Geometry check sheet. Reference: the model listing, model coordinates, mm. A direction names the side the tool comes from. Give positions to 0.01 mm unless a question says otherwise; leave off trailing zeros. Order: outer loops, then holes, each group sorted by start corner. A loop starts at its lowest first (then second) coordinate and runs counter-clockwise, first axis right, second up.
from build123d import *

# Parameters (mm, degrees)
BOSS_EXTRUDE1_DEPTH                                 = 15
TAP_DRILL_FOR_M6_TAP1_D                             = 5
CBORE_FOR_M6_HEX_SOCKET_HEAD_CAP_SCREW1_D           = 6.6
CBORE_FOR_M6_HEX_SOCKET_HEAD_CAP_SCREW1_CBORE_D     = 11
CBORE_FOR_M6_HEX_SOCKET_HEAD_CAP_SCREW1_CBORE_DEPTH = 6.4
CHAMFER1_SIZE                                       = 0.5


with BuildPart() as part:
    # Sketch1 → Boss-Extrude1 (new body)
    with BuildSketch(Plane.XY):
        with BuildLine():
            Line((2.914096072, -75.45920495), (9.914096072, -75.45920495))
            ThreePointArc((9.914096072, -75.45920495), (12.742523197, -74.287632074), (13.914096072, -71.45920495))
            Line((13.914096072, -71.45920495), (13.914096072, 14.148669163))
            ThreePointArc((13.914096072, 14.148669163), (14.675300747, 17.975503486), (16.84302826, 21.219736974))
            Line((16.84302826, 21.219736974), (18.985163884, 23.361872598))
            ThreePointArc((18.985163884, 23.361872598), (22.229397372, 25.529600111), (26.056231696, 26.290804786))
            Line((26.056231696, 26.290804786), (26.414096072, 26.290804786))
            ThreePointArc((26.414096072, 26.290804786), (32.914096072, 32.790804786), (26.414096072, 39.290804786))
            Line((26.414096072, 39.290804786), (20.671455385, 39.290804786))
            ThreePointArc((20.671455385, 39.290804786), (16.844621061, 38.529600111), (13.600387573, 36.361872598))
            Line((13.600387573, 36.361872598), (1.84302826, 24.604513285))
            ThreePointArc((1.84302826, 24.604513285), (-0.324699253, 21.360279797), (-1.085903928, 17.533445473))
            Line((-1.085903928, 17.533445473), (-1.085903928, -71.45920495))
            ThreePointArc((-1.085903928, -71.45920495), (0.085668947, -74.287632074), (2.914096072, -75.45920495))
        make_face()
    extrude(amount=BOSS_EXTRUDE1_DEPTH)

    # Tap Drill for M6 Tap1 (through all)
    with Locations(Plane.XY.offset(15)):
        with Locations((26.414096072, 32.790804786)):
            Hole(TAP_DRILL_FOR_M6_TAP1_D / 2)

    # CBORE for M6 Hex Socket Head Cap Screw1 (through all)
    with Locations(Plane(origin=(13.914096072, 0, 0), x_dir=(0, 0, -1), z_dir=(1, 0, 0))):
        with Locations((-7.5, -16.709195214), (-7.5, -61.709195214)):
            CounterBoreHole(CBORE_FOR_M6_HEX_SOCKET_HEAD_CAP_SCREW1_D / 2, CBORE_FOR_M6_HEX_SOCKET_HEAD_CAP_SCREW1_CBORE_D / 2, CBORE_FOR_M6_HEX_SOCKET_HEAD_CAP_SCREW1_CBORE_DEPTH)

    # Chamfer1
    chamfer1_edges = [part.edges().sort_by_distance(p)[0] for p in [
        (16.844621061, 38.529600111, 15),
        (7.721707916, 30.483192942, 15),
        (-0.324699253, 21.360279797, 15),
        (-1.085903928, -26.962879738, 15),
        (0.085668947, -74.287632074, 15),
        (6.414096072, -75.45920495, 15),
        (12.742523197, -74.287632074, 15),
        (13.914096072, -28.655267893, 15),
        (14.675300747, 17.975503486, 15),
        (17.914096072, 22.290804786, 15),
        (32.914096072, 32.790804786, 15),
        (22.229397372, 25.529600111, 15),
        (28.914096072, 32.790804786, 15),
        (26.235163884, 26.290804786, 15),
        (13.914096072, -61.709195214, 13),
        (13.914096072, -16.709195214, 13),
        (23.542775728, 39.290804786, 15),
    ]]
    chamfer(chamfer1_edges, length=CHAMFER1_SIZE)


solid = part.part
Item 1: Sectioned sample at B-B (z = 7.5). Give the number of separate pieces and of enclosed holes in the cut face, and give its area (3 significant figures).
Reported:
separate pieces: 3
enclosed holes: 1
area: 1,550 mm2
Item 2: Gauge pin test, flat ends, axial feed: pin 1 (9 mm diameter, centred on y = -16.71, z = 7.5, fed in from +X); pin 2 (8 mm diameter, centred on y = -5.5, z = 11.5, fed in from +X); pin 3 (5 mm diameter, centred on x = 4, z = 7.5, fed in from +Y). Record the tip position at first contact, or that the pin passes through.
Reported:
pin 1: stops at x = 7.51
pin 2: stops at x = 13.91
pin 3: stops at y = 29.26
Item 3: Draft check along Z on faces 1 (the conical face through (12.46, -74.06, 14.86)), 2 (the cylindrical face through (10.5, -12.1, 4.5)), 3 (the flat face through (7.804, 30.565, 7.148)). Enter one of: released by +Z, released by -Z, zero draft, split by the parting line, or undercut.
Reported:
face 1: released by +Z
face 2: undercut
face 3: zero draft
Item 4: Scan lines: L1, parallel to Y at x = 1, z = 10.5; L2, parallel to Y at x = 9, z = 3.75; L3, parallel to Y at x = 26.5, z = 7.5. Record each from-to range of solid material in increasing order.
Reported:
L1: y = -74.97 to -63.08, -60.33 to -18.08, -15.33 to 23.65
L2: y = -75.46 to -65.73, -57.69 to -20.73, -12.69 to 31.76
L3: y = 26.29 to 30.29, 35.29 to 39.29
Item 5: Set-up check for faces 4 (the flat face through (7.514, -65.3, 7.6)), 5 (the cylindrical face through (3.154, -58.437, 7.07)): record each of +Z, -Z, +X, -X, +Y, -Y from which the full face is reachable in a straight line by a thin tool's end or side.
Reported:
face 4: +X
face 5: +X, -X
Item 6: Sectioned sample at A-A (y = -7.5). Enter the section's corners in (x, z).
Reported:
outline: (-1.09, 0) - (13.91, 0) - (13.91, 14.5) - (13.41, 15) - (-0.59, 15) - (-1.09, 14.5) - close
